CAD build for the part. Positions are in the model's coordinates, mm. Round coordinates to 2 decimals unless told otherwise and drop trailing zeros. Write each loop counter-clockwise with the first axis right and the second up, starting at its lowest first coordinate (ties: lowest second). Pieces come first, ordered by that corner, then holes. Notation, with made-up numbers: (41.5, 8.25) - (55.5, 8.25) arc R13 cw to (55.5, 22.25) - close; hole circle Ø5 at (28, 59.5). An arc over 180 degrees is marked (long way). Answer in a Markdown table with one row per item.
```python
from build123d import *

# Parameters (mm, degrees)
SKETCH3_W           = 8.89
SKETCH3_H           = 3.175
BOSS_EXTRUDE2_DEPTH = 38.1
SKETCH4_R           = 1.4605
SKETCH4_R_2         = 1.27
CUT_EXTRUDE1_DEPTH  = 4.175


with BuildPart() as part:
    # Sketch3 → Boss-Extrude2 (new body)
    with BuildSketch(Plane(origin=(0, 0, 0), x_dir=(1, 0, 0), z_dir=(0, 1, 0))):
        with Locations((4.445, -5.1435)):
            Rectangle(SKETCH3_W, SKETCH3_H)
    extrude(amount=BOSS_EXTRUDE2_DEPTH)

    # Sketch4 → Cut-Extrude1 (cut, through all)
    with BuildSketch(Plane.XY.offset(6.731)):
        with Locations((4.445, 33.02)):
            Circle(SKETCH4_R)
        with Locations((4.445, 12.169083682)):
            Circle(SKETCH4_R_2)
        with Locations((4.445, 22.329083682)):
            Circle(SKETCH4_R_2)
    extrude(amount=-CUT_EXTRUDE1_DEPTH, mode=Mode.SUBTRACT)


solid = part.part
```
Q1. Pull direction Y, two halves, no side cores. Call faces 1 (the cylindrical face through (4.28, 23.59, 5.17)), 2 (the flat face through (4, 19, 6.731)), 3 (the flat face through (4, 0, 5)): released by +Y, released by -Y, zero draft, split by the parting line, or undercut.
Computed:
| item | result |
|---|---|
| face 1 | undercut |
| face 2 | zero draft |
| face 3 | released by -Y |
Q2. Saw through at C-C on z = 6. List the corners of the cut face in (x, y) (1 decimal), then the cut area to 3 significant figures.
Computed:
| item | result |
|---|---|
| outline | (0, 0) - (8.9, 0) - (8.9, 38.1) - (0, 38.1) - close; hole circle Ø2.9 at (4.4, 33); hole circle Ø2.5 at (4.4, 12.2); hole circle Ø2.5 at (4.4, 22.3) |
| area | 322 mm2 |
Q3. Drill centre lines: line 1 (Y direction, x = 4.5, z = 4.4); line 2 (Y direction, x = 5.5, z = 4.35); line 3 (Y direction, x = 5.75, z = 4.75). Where is each one in solid material? Low to high.
Computed:
| item | result |
|---|---|
| line 1 | y = 0 to 10.9, 13.44 to 21.06, 23.6 to 31.56, 34.48 to 38.1 |
| line 2 | y = 0 to 11.46, 12.88 to 21.62, 23.04 to 32.01, 34.03 to 38.1 |
| line 3 | y = 0 to 32.36, 33.68 to 38.1 |
Q4. Saw through at B-B on x = 4.5. List the corners of the cut face in (y, z), then the cut area to 3 significant figures.
Computed:
| item | result |
|---|---|
| outline | (0, 3.56) - (10.9, 3.56) - (10.9, 6.73) - (0, 6.73) - close; (13.44, 3.56) - (21.06, 3.56) - (21.06, 6.73) - (13.44, 6.73) - close; (23.6, 3.56) - (31.56, 3.56) - (31.56, 6.73) - (23.6, 6.73) - close; (34.48, 3.56) - (38.1, 3.56) - (38.1, 6.73) - (34.48, 6.73) - close |
| area | 95.6 mm2 |
Q5. Saw through at A-A on y = 33.02. List the corners of the cut face in (x, z), then the cut area to 3 significant figures.
Computed:
| item | result |
|---|---|
| outline | (0, 3.56) - (2.98, 3.56) - (2.98, 6.73) - (0, 6.73) - close; (5.91, 3.56) - (8.89, 3.56) - (8.89, 6.73) - (5.91, 6.73) - close |
| area | 19.0 mm2 |
